```python
from build123d import *

# Parameters (mm, degrees)
SKETCH1_R           = 11
SKETCH1_R_2         = 10
BOSS_EXTRUDE3_DEPTH = 10


with BuildPart() as part:
    # Sketch1 → Boss-Extrude3 (new body)
    # profile 1 of 6: a face of its own
    with BuildSketch(Plane(origin=(0, 0, 0), x_dir=(1, 0, 0), z_dir=(0, 1, 0))):
        Circle(SKETCH1_R)
        with Locations(Location((0, 0, 0), (0, 0, 270))):
            Circle(SKETCH1_R_2, mode=Mode.SUBTRACT)
    # profile 2 of 6: a face of its own
    with BuildSketch(Plane(origin=(0, 0, 0), x_dir=(1, 0, 0), z_dir=(0, 1, 0))):
        with BuildLine():
            ThreePointArc((-9.526279142, -5.500000519), (-11, -3e-09), (-9.526279145, 5.500000513))
            Line((-9.526279145, 5.500000513), (-12.701705922, 0))
            Line((-12.701705922, 0), (-9.526279142, -5.500000519))
        make_face()
    # profile 3 of 6: a face of its own
    with BuildSketch(Plane(origin=(0, 0, 0), x_dir=(1, 0, 0), z_dir=(0, 1, 0))):
        with BuildLine():
            Line((-6.350852961, -11), (5.6e-08, -11))
            ThreePointArc((5.6e-08, -11), (-5.499999716, -9.526279605), (-9.526279142, -5.500000519))
            Line((-9.526279142, -5.500000519), (-6.350852961, -11))
        make_face()
    # profile 4 of 6: a face of its own
    with BuildSketch(Plane(origin=(0, 0, 0), x_dir=(1, 0, 0), z_dir=(0, 1, 0))):
        with BuildLine():
            Line((6.350852961, -11), (9.526279442, -5.5))
            ThreePointArc((9.526279442, -5.5), (5.500000024, -9.526279428), (5.6e-08, -11))
            Line((5.6e-08, -11), (6.350852961, -11))
        make_face()
    # profile 5 of 6: a face of its own
    with BuildSketch(Plane(origin=(0, 0, 0), x_dir=(1, 0, 0), z_dir=(0, 1, 0))):
        with BuildLine():
            ThreePointArc((0, 11), (5.5, 9.526279442), (9.526279442, 5.5))
            Line((9.526279442, 5.5), (6.350852961, 11))
            Line((6.350852961, 11), (0, 11))
        make_face()
    # profile 6 of 6: a face of its own
    with BuildSketch(Plane(origin=(0, 0, 0), x_dir=(1, 0, 0), z_dir=(0, 1, 0))):
        with BuildLine():
            ThreePointArc((-9.526279145, 5.500000513), (-5.499999743, 9.52627959), (0, 11))
            Line((0, 11), (-6.350852961, 11))
            Line((-6.350852961, 11), (-9.526279145, 5.500000513))
        make_face()
    extrude(amount=BOSS_EXTRUDE3_DEPTH)


solid = part.part
```
For this review, take the finished solid that the model builds, in its own axes (mm). Coordinates: 2 decimals unless noted, no trailing zeros. Loops run counter-clockwise (first coordinate to the right, second up) from the corner with the lowest first, then second, coordinate; pieces in that order, holes last.
1. Add section D-D, the plane x = -11. Give the boundary of the cut face in (y, z).
2. Add section A-A, the plane x = 0. Give the boundary of the cut face in (y, z), then the cut area to 3 significant figures.
3. Add section B-B, the plane y = 6.5. Give the boundary of the cut face in (x, z), then the cut area to 3 significant figures.
4. Mouldability with a two-part tool opening along Z and no side actions: class faces 1 (the flat face through (0, 5, -11)), 2 (the cylindrical face through (-9.76, 4.93, -2.17)), 3 (the cylindrical face through (11, 5, 0)), 4 (the flat face through (-10, 10, -2)) as +Z half, -Z half, draft (parallel to the pull), parting line (faces both ways), or undercut.
5. For line 1 (Z direction, x = -4.75, y = 3.75); line 2 (X direction, y = 2.75, z = 5.25); line 3 (Z direction, x = -0.5, y = 2.75), list the stretches that pass through material, from the lowest coordinate up.
6. Insertion check: P1, Ø4, axis at y = 3.5, z = 6.5, coming from the +X side. The pin has a flat end and moves straight along its axis. Give the tip position at first contact, or say it passes through.
7. Add section C-C, the plane z = 2. Give the boundary of the cut face in (x, y), then the cut area to 3 significant figures.
Result:
1. outline: (0, -2.95) - (10, -2.95) - (10, 2.95) - (0, 2.95) - close
2. outline: (0, -11) - (10, -11) - (10, -10) - (0, -10) - close; (0, 10) - (10, 10) - (10, 11) - (0, 11) - close
2. area: 20.0 mm2
3. outline: (-12.7, 0) - (-6.35, -11) - (6.35, -11) - (9.53, -5.5) arc R11 ccw to (9.53, 5.5) - (6.35, 11) - (-6.35, 11) - close; hole circle Ø20 at (0, 0)
3. area: 98.5 mm2
4. face 1: -Z half
4. face 2: undercut
4. face 3: parting line
4. face 4: draft
5. line 1: z = -11 to -8.8, 8.8 to 11
5. line 2: x = -9.67 to -8.51, 8.51 to 9.67
5. line 3: z = -11 to -9.99, 9.99 to 11
6. P1: stops at x = 10.04
7. outline: (-11.55, 0) - (-9.8, 0) - (-9.8, 10) - (-11.55, 10) - close; (9.8, 0) - (10.82, 0) - (10.82, 10) - (9.8, 10) - close
7. area: 27.7 mm2
